Autodesk Inventor part; units mm, degrees
ref_plane "YZ Plane" through (0, 0, 0) normal (1, 0, 0) x (0, 1, 0)
ref_plane "XZ Plane" through (0, 0, 0) normal (0, 1, 0) x (-1, 0, 0)
ref_plane "XY Plane" through (0, 0, 0) normal (0, 0, 1) x (1, 0, 0)
sketch "Sketch1" plane through (0, 0, 0) normal (0, 1, 0) x (-1, 0, 0)
  line L0 (0, 0) -> (0, 50.8)
  line L1 (0, 50.8) -> (50.8, 50.8)
  line L2 (50.8, 50.8) -> (50.8, 47.625)
  line L3 (50.8, 47.625) -> (3.175, 47.625)
  line L4 (3.175, 47.625) -> (3.175, 0)
  line L5 (3.175, 0) -> (0, 0)
  dimension "d0" = 50.8
  dimension "d1" = 50.8
  dimension "d2" = 3.175
  dimension "d3" = 47.625
  dimension "d4" = 47.625
extrude "Extrusion1" add sketch "Sketch1" along normal blind 50.8
sketch "Sketch3" plane through (-3.175, 0, 0) normal (-1, 0, 0) x (0, 0, 1)
  circle A0 centre (23.8125, 25.4) radius 25.4 construction
  line L0 (0, 50.8) -> (47.625, 50.8)
  line L1 (0, 0) -> (0, 50.8)
  circle A1 centre (6.3119, 43.8089) radius 2.032
  circle A2 centre (41.3131, 6.9911) radius 2.032
  line L2 (0, 0) -> (50.8, 0)
  line L3 (23.8125, 0) -> (23.8125, 50.8) construction
  line L4 (50.8, 50.8) -> (0, 50.8)
  circle A3 centre (23.8125, 25.4) radius 9.525
  dimension "d12" = 50.8
  dimension "d13" = 25.4
  dimension "d14" = 23.8125
  dimension "d15" = 4.064
  dimension "d16" = 4.064
  dimension "d17" = 17.5006
  dimension "d18" = 17.5006
  dimension "d19" = 19.05
extrude "Extrusion2" cut sketch "Sketch3" against normal blind 3.175
properties part number "BAG motor bracket" material "Aluminum 6061"
CAD build for the part. Positions are in the model's coordinates, mm. A direction names the side the tool comes from. Round coordinates to 2 decimals unless told otherwise and drop trailing zeros. Write each loop counter-clockwise with the first axis right and the second up, starting at its lowest first coordinate (ties: lowest second). Pieces come first, ordered by that corner, then holes. Notation, with made-up numbers: (39.25, -8.75) -> (73.25, -8.75) arc R29 cw to (73.25, 28.25) -> close; hole circle Ø5 at (73, -0.5). An arc over 180 degrees is marked (long way). Answer in a Markdown table with one row per item. Add a question column.
Item 1: Saw through at A-A, the plane y = 25.4. Write the cut outline in (x, z) (1 decimal).
Item 2: Drop flat-ended pins along their axis: pin 1 Ø24 at (y, z) = (24, 18) entering from -X (3 decimals); pin 2 Ø2 at (x, y) = (-5.5, 9.5) entering from -Z (3 decimals). Give the stop position or say it passes through.
Item 3: Drill centre lines: line 1 (Z direction, x = -2, y = 25); line 2 (X direction, y = 38.5, z = 14.5) (3 decimals); line 3 (Z direction, x = -15.5, y = 48.5) (3 decimals). Where is each one in solid material? Low to high. Write a range as from..to.
Item 4: Saw through at B-B, the plane z = 25.5. Write the cut outline in (x, y) (3 decimals), then the cut area to 3 significant figures.
Item 5: Saw through at D-D, the plane y = 11.5. Write the cut outline in (x, z) (3 decimals), then the cut area to 4 significant figures.
Item 6: Saw through at C-C, the plane x = -29. Write the cut outline in (y, z) (3 decimals), then the cut area to 3 significant figures.
Item 7: Which spindle directions (+Z, -Z, +X, -X, +Y, -Y) get a long thin tool onto all of the face, cutting with end or side? Do faces 1 (the face through (-1.61, 7.6, 43.25)), 2 (the face through (-3.175, 25, 14)). Say none if no direction does.
Item 8: Mould opens along Y. For faces 3 (the face through (-25, 25, 50.8)), 4 (the face through (-1.61, 45.18, 4.81)), 5 (the face through (-3, 50.8, 37)) say: pulls with the +Y half, pulls with the -Y half, needs draft (parallel to the pull), parting line crosses it, or undercut.
Findings below:
| question | item | result |
|---|---|---|
| 1 | outline | (-50.8, 47.6) -> (-3.2, 47.6) -> (-3.2, 33.3) -> (0, 33.3) -> (0, 50.8) -> (-50.8, 50.8) -> close; (-3.2, 0) -> (0, 0) -> (0, 14.3) -> (-3.2, 14.3) -> close |
| 2 | pin 1 | stops at x = -3.175 |
| 2 | pin 2 | stops at z = 47.625 |
| 3 | line 1 | z = 0..14.3, 33.33..50.8 |
| 3 | line 2 | x = -3.175..0 |
| 3 | line 3 | z = 47.625..50.8 |
| 4 | outline | (-3.175, 0) -> (0, 0) -> (0, 16.026) -> (-3.175, 16.026) -> close; (-3.175, 34.774) -> (0, 34.774) -> (0, 50.8) -> (-3.175, 50.8) -> close |
| 4 | area | 102 mm^2 |
| 5 | outline | (-50.8, 47.625) -> (-3.175, 47.625) -> (-3.175, 0) -> (0, 0) -> (0, 50.8) -> (-50.8, 50.8) -> close |
| 5 | area | 312.5 mm^2 |
| 6 | outline | (0, 47.625) -> (50.8, 47.625) -> (50.8, 50.8) -> (0, 50.8) -> close |
| 6 | area | 161 mm^2 |
| 7 | face 1 | +X, -X |
| 7 | face 2 | -Z, -X, +Y, -Y |
| 8 | face 3 | needs draft |
| 8 | face 4 | undercut |
| 8 | face 5 | pulls with the +Y half |
